Build history of the part. All positions in model axes, mm. Round coordinates to 2 decimals unless told otherwise and drop trailing zeros. Write each loop counter-clockwise with the first axis right and the second up, starting at its lowest first coordinate (ties: lowest second). Pieces come first, ordered by that corner, then holes. Notation, with made-up numbers: (41.25, 71.5) -> (66.25, 71.5) arc R33 cw to (66.25, 103.5) -> close; hole circle Ø10 at (81.25, 86). An arc over 180 degrees is marked (long way). Answer as CSV lines item,"result".
from build123d import *

# Parameters (mm, degrees)
SKETCH1_R           = 1.75
BOSS_EXTRUDE1_DEPTH = 3


with BuildPart() as part:
    # Sketch1 → Boss-Extrude1 (new body)
    with BuildSketch(Plane.XY):
        with BuildLine():
            Line((-146, 333.999999944), (146, 333.999999944))
            ThreePointArc((146, 333.999999944), (148.121320344, 333.121320287), (149, 330.999999944))
            Line((149, 330.999999944), (149, 226.999999944))
            ThreePointArc((149, 226.999999944), (148.121320344, 224.8786796), (146, 223.999999944))
            Line((146, 223.999999944), (129.53838912, 223.999999944))
            Line((129.53838912, 223.999999944), (129.53838912, 219))
            Line((129.53838912, 219), (73.53838912, 219))
            Line((73.53838912, 219), (28.510237275, 219))
            Line((28.510237275, 219), (28.510237275, 246.944274273))
            ThreePointArc((28.510237275, 246.944274273), (28.803130494, 247.651381054), (29.510237275, 247.944274273))
            Line((29.510237275, 247.944274273), (38.432325919, 247.944274273))
            ThreePointArc((38.432325919, 247.944274273), (39.846539481, 248.530060711), (40.432325919, 249.944274273))
            Line((40.432325919, 249.944274273), (40.432325919, 327.952168393))
            ThreePointArc((40.432325919, 327.952168393), (40.096133825, 328.763807906), (39.284494312, 329.1))
            Line((39.284494312, 329.1), (-38.419842474, 329.1))
            ThreePointArc((-38.419842474, 329.1), (-39.231481987, 328.763807906), (-39.567674081, 327.952168393))
            Line((-39.567674081, 327.952168393), (-39.567674081, 248.944274273))
            ThreePointArc((-39.567674081, 248.944274273), (-39.274780862, 248.237167492), (-38.567674081, 247.944274273))
            Line((-38.567674081, 247.944274273), (-29.469288178, 247.944274273))
            ThreePointArc((-29.469288178, 247.944274273), (-28.762181396, 247.651381054), (-28.469288178, 246.944274273))
            Line((-28.469288178, 246.944274273), (-28.469288178, 218.999999943))
            Line((-28.469288178, 218.999999943), (-70, 218.999999943))
            Line((-70, 218.999999943), (-126, 218.999999943))
            Line((-126, 218.999999943), (-126, 223.999999944))
            Line((-126, 223.999999944), (-146, 223.999999944))
            ThreePointArc((-146, 223.999999944), (-148.121320343, 224.8786796), (-149, 226.999999944))
            Line((-149, 226.999999944), (-149, 330.999999944))
            ThreePointArc((-149, 330.999999944), (-148.121320343, 333.121320287), (-146, 333.999999944))
        make_face()
        with Locations((-136, 321.999999944)):
            Circle(SKETCH1_R, mode=Mode.SUBTRACT)
        with Locations((-136, 235.999999944)):
            Circle(SKETCH1_R, mode=Mode.SUBTRACT)
        with Locations(Location((136, 235.999999944, 0), (0, 0, 180))):
            Circle(SKETCH1_R, mode=Mode.SUBTRACT)
        with Locations(Location((136, 321.999999944, 0), (0, 0, 180))):
            Circle(SKETCH1_R, mode=Mode.SUBTRACT)
        with Locations((108.5, 311.539999944)):
            Circle(SKETCH1_R, mode=Mode.SUBTRACT)
        with Locations((108.5, 300.499999944)):
            Circle(SKETCH1_R, mode=Mode.SUBTRACT)
        with Locations((108.5, 281.539999944)):
            Circle(SKETCH1_R, mode=Mode.SUBTRACT)
        with Locations((108.5, 270.499999944)):
            Circle(SKETCH1_R, mode=Mode.SUBTRACT)
        with Locations((108.5, 251.539999944)):
            Circle(SKETCH1_R, mode=Mode.SUBTRACT)
        with Locations((108.5, 240.499999944)):
            Circle(SKETCH1_R, mode=Mode.SUBTRACT)
        with BuildLine():
            Line((52.97092131, 313.1), (77.97092131, 313.1))
            ThreePointArc((77.97092131, 313.1), (78.678028091, 312.807106781), (78.97092131, 312.1))
            Line((78.97092131, 312.1), (78.97092131, 272.1))
            ThreePointArc((78.97092131, 272.1), (78.678028091, 271.392893219), (77.97092131, 271.1))
            Line((77.97092131, 271.1), (52.97092131, 271.1))
            ThreePointArc((52.97092131, 271.1), (52.263814529, 271.392893219), (51.97092131, 272.1))
            Line((51.97092131, 272.1), (51.97092131, 312.1))
            ThreePointArc((51.97092131, 312.1), (52.263814529, 312.807106781), (52.97092131, 313.1))
        make_face(mode=Mode.SUBTRACT)
    extrude(amount=BOSS_EXTRUDE1_DEPTH)


solid = part.part
1. Cut at A-A, the plane y = 275. Write the cut outline in (x, z).
Results found:
outline,"(-149, 0) -> (-39.57, 0) -> (-39.57, 3) -> (-149, 3) -> close; (40.43, 0) -> (51.97, 0) -> (51.97, 3) -> (40.43, 3) -> close; (78.97, 0) -> (149, 0) -> (149, 3) -> (78.97, 3) -> close"
2. Drop a flat-ended pin along its axis: pin 1 Ø1 at (x, z) = (-15, 2) entering from -Y. Give the stop position or say it passes through.
Results found:
pin 1,"stops at y = 329.1"
3. Cut at B-B, the plane z = 1.55. Count the separate pieces of the cut face and the enclosed holes in it, then the cut area to 3 significant figures.
Results found:
separate pieces,"1"
enclosed holes,"11"
area,"24,700 mm2"
4. Probe line 1 along X through (y, z) = (236, 1.3); line 2 along X through (y, z) = (285.5, 0.4); line 3 along X through (y, z) = (322, 1.85). List the from-to ranges inside material, lowest first.
Results found:
line 1,"x = -149 to -137.75, -134.25 to -28.47, 28.51 to 134.25, 137.75 to 149"
line 2,"x = -149 to -39.57, 40.43 to 51.97, 78.97 to 149"
line 3,"x = -149 to -137.75, -134.25 to -39.57, 40.43 to 134.25, 137.75 to 149"
5. Cut at C-C, the plane x = 22. Write the cut outline in (y, z), then the cut area to 3 significant figures.
Results found:
outline,"(329.1, 0) -> (334, 0) -> (334, 3) -> (329.1, 3) -> close"
area,"14.7 mm2"
